Check sheet for the drawn part. Datum: minimum x, y, z corner. Units: mm. A direction names the side the tool comes from. Round coordinates to 2 decimals unless told otherwise and drop trailing zeros. Write each loop counter-clockwise with the first axis right and the second up, starting at its lowest first coordinate (ties: lowest second). Pieces come first, ordered by that corner, then holes. Notation, with made-up numbers: M 64.5,26 L 93.5,26 A15 cw 93.5,38 Z; hole C 80.5,49 d1. An arc over 180 degrees is marked long. Use a Markdown table: item, result.
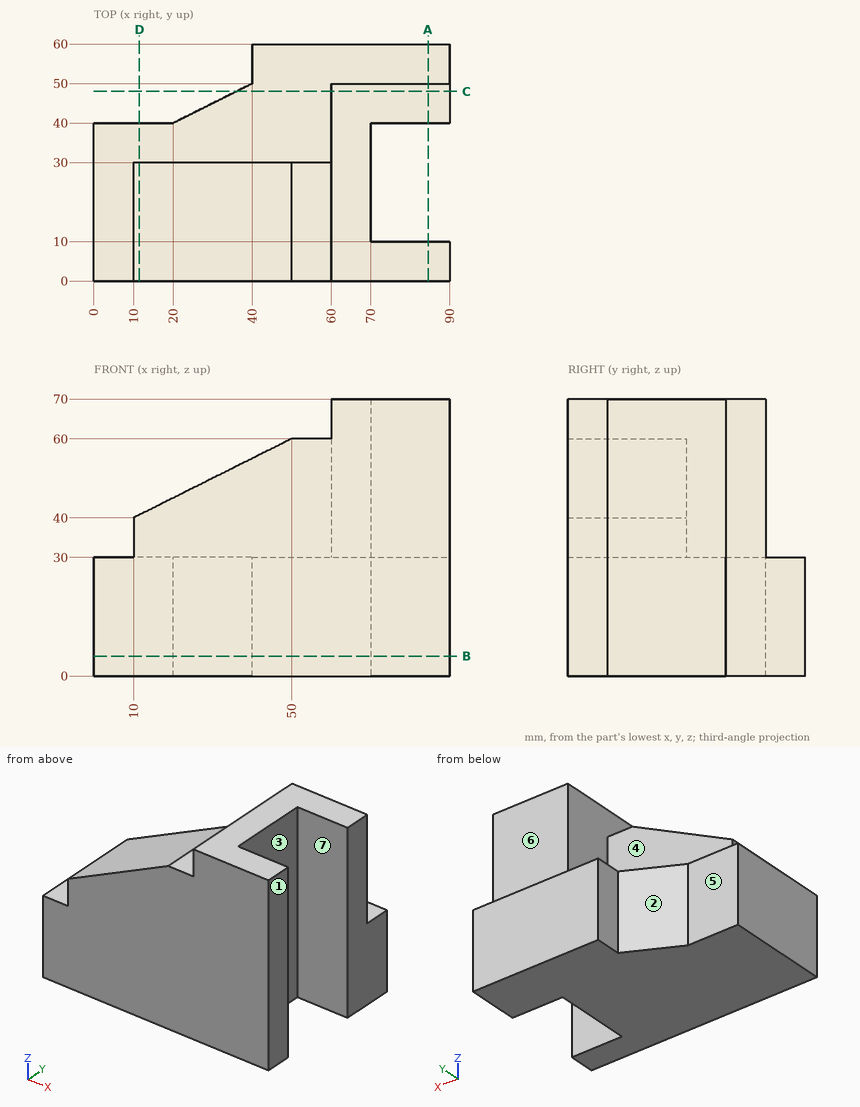
Item 1: Cross-section at D-D, the plane x = 11.5. Record the cut outline in (y, z).
Outcome:
| item | result |
|---|---|
| outline | M 0,0 L 40,0 L 40,30 L 30,30 L 30,40.75 L 0,40.75 Z |
Item 2: Go/stop test with flat-tipped pins: pin 1 (24 mm diameter, centred on x = 26.5, z = 43, fed in from +Y); pin 2 (5 mm diameter, centred on y = 57, z = 10.5, fed in from -X); pin 3 (4 mm diameter, centred on y = 22, z = 47.5, fed in from +X). Record where each tip stops, or that it passes through.
Outcome:
| item | result |
|---|---|
| pin 1 | stops at y = 30 |
| pin 2 | stops at x = 40 |
| pin 3 | stops at x = 70 |
Item 3: Cross-section at C-C, the plane y = 48. Record the cut outline in (x, z).
Outcome:
| item | result |
|---|---|
| outline | M 36,0 L 90,0 L 90,70 L 60,70 L 60,30 L 36,30 Z |
Item 4: Material ranges on line 1 along Y through (x, z) = (70.5, 51); line 2 along X through (y, z) = (31.5, 32); line 3 along Z through (x, y) = (13, 34), recorded low to high. Write a range as from..to.
Outcome:
| item | result |
|---|---|
| line 1 | y = 0..10, 40..50 |
| line 2 | x = 60..70 |
| line 3 | z = 0..30 |
Item 5: Cross-section at B-B, the plane z = 5. Record the cut outline in (x, y), and give its area (3 significant figures).
Outcome:
| item | result |
|---|---|
| outline | M 0,0 L 90,0 L 90,10 L 70,10 L 70,40 L 90,40 L 90,60 L 40,60 L 40,50 L 20,40 L 0,40 Z |
| area | 4,100 mm2 |
Item 6: Cross-section at A-A, the plane x = 84.5. Record the cut outline in (y, z).
Outcome:
| item | result |
|---|---|
| outline | M 0,0 L 10,0 L 10,70 L 0,70 Z; M 40,0 L 60,0 L 60,30 L 50,30 L 50,70 L 40,70 Z |
Item 7: Mould release check, pull along Y, two halves, no side actions. Record for the marked faces 1, 2 and 3: +Y half, -Y half, draft (parallel to the pull), parting line (faces both ways), or undercut.
Outcome:
| item | result |
|---|---|
| face 1 | draft |
| face 2 | +Y half |
| face 3 | undercut |
Item 8: Access from +Z, -Z, +X, -X, +Y, -Y to the whole of each face (thin tool, end or side, straight path). Record for the marked faces 4, 5, 6 and 7.
Outcome:
| item | result |
|---|---|
| face 4 | +Z, -X, +Y |
| face 5 | +Z, -Z, -X, +Y |
| face 6 | +Z, +X, -X, +Y |
| face 7 | +Z, -Z, +X |
